from build123d import *

# Parameters (mm, degrees)
F0_R     = 12.7
F1_DEPTH = 9.525
F3_D     = 6.35
F3_DEPTH = 5.08
F3_TIP   = 1.9077324654
F5_DEPTH = 25.4


# Not quite as in the source:
# - a feature names something its author has since deleted; it is built from what else it names


with BuildPart() as f1:
    # F0 (on Top) → F1 (new body)
    with BuildSketch(Plane.XY):
        Circle(F0_R)
    extrude(amount=F1_DEPTH)

    # F3
    with Locations(Plane.XY.offset(9.525)):
        with Locations((0, 0)):
            Hole(F3_D / 2, depth=F3_DEPTH)
            with Locations((0, 0, -(F3_DEPTH + F3_TIP / 2))):  # 118° drill point
                Cone(0, F3_D / 2, F3_TIP, mode=Mode.SUBTRACT)

    # F4 (on face) → F5 (cut)
    with BuildSketch(Plane.XY.offset(9.525)):
        with BuildLine():
            Line((19.05, -9.525), (19.05, 9.525))
            Line((19.05, 9.525), (8.4002604126, 9.525))
            ThreePointArc((8.4002604126, 9.525), (11.5752604126, 5.2252604126), (12.7, 0))
            ThreePointArc((12.7, 0), (11.5752604126, -5.2252604126), (8.4002604126, -9.525))
            Line((8.4002604126, -9.525), (19.05, -9.525))
        make_face()
        with BuildLine():
            ThreePointArc((-8.4002604126, -9.525), (-12.7, 0), (-8.4002604126, 9.525))
            Line((-8.4002604126, 9.525), (-19.05, 9.525))
            Line((-19.05, 9.525), (-19.05, -9.525))
            Line((-19.05, -9.525), (-8.4002604126, -9.525))
        make_face()
        with BuildLine():
            ThreePointArc((-8.4002604126, -9.525), (0, -12.7), (8.4002604126, -9.525))
            Line((8.4002604126, -9.525), (-8.4002604126, -9.525))
        make_face()
        with BuildLine():
            Line((-8.4002604126, 9.525), (8.4002604126, 9.525))
            ThreePointArc((8.4002604126, 9.525), (0, 12.7), (-8.4002604126, 9.525))
        make_face()
    extrude(amount=-F5_DEPTH, mode=Mode.SUBTRACT)


solid = f1.part
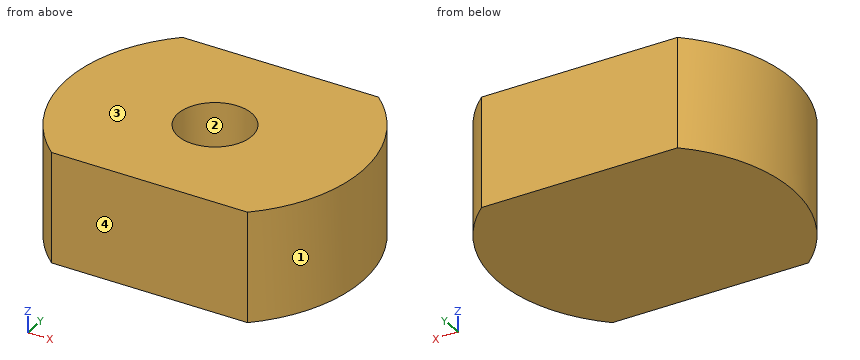
Could you check a few things on this model? Use its own coordinates, in mm. Face numbers are marked on the shaded views. Coordinates: 2 decimals unless noted, no trailing zeros. Order: outer loops, then holes, each group sorted by start corner. A loop starts at its lowest first (then second) coordinate and runs counter-clockwise, first axis right, second up. Notation, with made-up numbers: (45, 69.25) - (51, 69.25) arc R10 ccw to (51, 78.25) - close; hole circle Ø1 at (-12, 34.25). An arc over 180 degrees is marked (long way). Answer in a Markdown table with one row per item. Add a question column.
(1) If we section it at A-A, the plane z = 6.25: Please give me the cut outline in (x, y) (3 decimals).
(2) Will these pins go through, and if not, where does the flat tip stop? pin 1 (1 mm diameter, centred on y = -2, z = 7, fed in from -X); pin 2 (1.5 mm diameter, centred on y = 7, z = 5, fed in from +X); pin 3 (1.5 mm diameter, centred on y = 3.5, z = 3.5, fed in from +X).
(3) If we mould it in two halves opening along Y, with no side actions, what happens to the marked faces 1, 2, 3 and 4? For each: released by +Y, released by -Y, zero draft, split by the parting line, or undercut.
(4) I need wall thicknesses on L1, parallel to X at y = 0, z = 6.65 (3 decimals); L2, parallel to Y at x = 0, z = 5.7 (3 decimals); L3, parallel to Y at x = -2.25, z = 6.5 (3 decimals). Which ranges of each line are inside material? Lowest first, please.
(5) If we section it at C-C, the plane y = -7.5: Please give me the cut outline in (x, z) (3 decimals), then the cut area to 3 significant figures.
(6) If we section it at B-B, the plane z = 1.75: Please give me the cut outline in (x, y) (3 decimals).
Results are:
| question | item | result |
|---|---|---|
| 1 | outline | (-8.4, -9.525) - (8.4, -9.525) arc R12.7 ccw to (8.4, 9.525) - (-8.4, 9.525) arc R12.7 ccw to start; hole circle Ø6.35 at (0, 0) |
| 2 | pin 1 | stops at x = -12.61 |
| 2 | pin 2 | stops at x = 11.06 |
| 2 | pin 3 | stops at x = 12.4 |
| 3 | face 1 | split by the parting line |
| 3 | face 2 | undercut |
| 3 | face 3 | zero draft |
| 3 | face 4 | released by -Y |
| 4 | L1 | x = -12.7 to -3.175, 3.175 to 12.7 |
| 4 | L2 | y = -9.525 to -3.175, 3.175 to 9.525 |
| 4 | L3 | y = -9.525 to -2.24, 2.24 to 9.525 |
| 5 | outline | (-10.249, 0) - (10.249, 0) - (10.249, 9.525) - (-10.249, 9.525) - close |
| 5 | area | 195 mm2 |
| 6 | outline | (-8.4, -9.525) - (8.4, -9.525) arc R12.7 ccw to (8.4, 9.525) - (-8.4, 9.525) arc R12.7 ccw to start |
